```python
from build123d import *

# Parameters (mm, degrees)
PAD002_DEPTH = 2.1
SKETCH003_R  = 1
PAD003_DEPTH = 14.3
SKETCH004_R  = 2.05
PAD004_DEPTH = 2.1
PAD005_DEPTH = 8.5


with BuildPart() as part:
    # Sketch002 → Pad002 (new body)
    with BuildSketch(Plane.XZ.offset(-2.5)):
        Polygon((-56.845299, -2), (-55.690599, 0), (-56.845299, 2), (-59.154701, 2), (-60.309401, 0), (-59.154701, -2), align=None)
    extrude(amount=PAD002_DEPTH)

    # Sketch003 (on Face8 of Pad002) → Pad003 (join)
    with BuildSketch(Plane.XZ.offset(-0.4)):
        with Locations((-58, 0)):
            Circle(SKETCH003_R)
    extrude(amount=PAD003_DEPTH)

    # Sketch004 (on Face10 of Pad003) → Pad004 (join)
    with BuildSketch(Plane.XZ.offset(13.9)):
        with Locations((-58, 0)):
            Circle(SKETCH004_R)
    extrude(amount=PAD004_DEPTH)

    # Sketch005 → Pad005 (join)
    with BuildSketch(Plane.XZ.offset(2.5)):
        with BuildLine():
            Line((-68, 10), (-54, 10))
            Line((-54, 10), (-54, 0))
            ThreePointArc((-58, -4), (-55.171573, -2.828427), (-54, 0))
            Line((-58, -4), (-68, -4))
            Line((-68, -4), (-68, 10))
        make_face()
    extrude(amount=PAD005_DEPTH)


solid = part.part
```
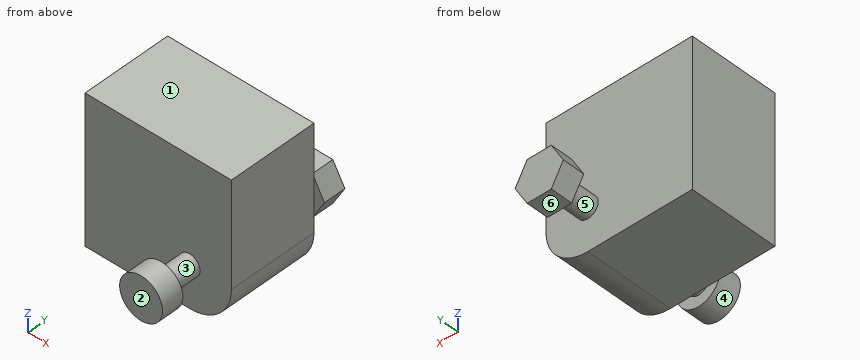
Build history of the part. All positions in model axes, mm. Face numbers are marked on the shaded views. A direction names the side the tool comes from. Give positions to 0.01 mm unless a question says otherwise; leave off trailing zeros. Loops run counter-clockwise (first coordinate to the right, second up) from the corner with the lowest first, then second, coordinate; pieces in that order, holes last.
1) Band-saw the part on A-A on y = -7. List the corners of the cut face in (x, z), then the cut area to 3 significant figures.
Values follow:
outline: (-68, -4) - (-58, -4) arc R4 ccw to (-54, 0) - (-54, 10) - (-68, 10) - close
area: 193 mm2
2) Band-saw the part on C-C on x = -65.5. List the corners of the cut face in (y, z), then the cut area to 3 significant figures.
Values follow:
outline: (-11, -4) - (-2.5, -4) - (-2.5, 10) - (-11, 10) - close
area: 119 mm2
3) Band-saw the part on B-B on z = 6. List the corners of the cut face in (x, y), then the cut area to 3 significant figures.
Values follow:
outline: (-68, -11) - (-54, -11) - (-54, -2.5) - (-68, -2.5) - close
area: 119 mm2
4) Two-plate mould, pull along Y, no slides. Class the marked faces 1, 2 and 3: released by +Y, released by -Y, zero draft, split by the parting line, or undercut.
Values follow:
face 1: zero draft
face 2: released by -Y
face 3: undercut
5) Probe line 1 along Y through (x, z) = (-62.5, 1.5); line 2 along Z through (x, y) = (-55, -5.5); line 3 along X through (y, z) = (-0.5, 0.25). List the from-to ranges inside material, lowest first.
Values follow:
line 1: y = -11 to -2.5
line 2: z = -2.65 to 10
line 3: x = -58.97 to -57.03
6) Drop flat-ended pins along their axis: P1, Ø1.5, axis at x = -55.5, y = -10, coming from the -Z side; P2, Ø4, axis at x = -64, z = 2, coming from the -Y side; P3, Ø1.7, axis at x = -58.5, y = 1.5, coming from the -Z side. Give the stop position or say it passes through.
Values follow:
P1: stops at z = -3.6
P2: stops at y = -11
P3: stops at z = -2
7) 3-axis set-ups, long thin cutter, end or side, ignore diameter. For the marked faces 4, 5 and 6: which of +Z, -Z, +X, -X, +Y, -Y reach the whole face in a straight line?
Values follow:
face 4: -Y
face 5: none
face 6: -Z, +X, -X, +Y
8) Band-saw the part on D-D on z = -0.25. List the corners of the cut face in (x, y), then the cut area to 3 significant figures.
Values follow:
outline: (-68, -11) - (-58.97, -11) - (-58.97, -13.9) - (-60.03, -13.9) - (-60.03, -16) - (-55.97, -16) - (-55.97, -13.9) - (-57.03, -13.9) - (-57.03, -11) - (-54.01, -11) - (-54.01, -2.5) - (-57.03, -2.5) - (-57.03, 0.4) - (-55.83, 0.4) - (-55.83, 2.5) - (-60.17, 2.5) - (-60.17, 0.4) - (-58.97, 0.4) - (-58.97, -2.5) - (-68, -2.5) - close
area: 148 mm2
